Source: CAD feature listing. Evaluate the final solid. Frame: model axes, mm. Face numbers are marked on the shaded views. A direction names the side the tool comes from. Coordinates: 2 decimals unless noted, no trailing zeros. Write each loop counter-clockwise with the first axis right and the second up, starting at its lowest first coordinate (ties: lowest second). Pieces come first, ordered by that corner, then holes. Notation, with made-up numbers: (70.5, 63.25) - (87.5, 63.25) arc R21 cw to (87.5, 97.25) - close; hole circle Ø10 at (74.5, -18). An arc over 180 degrees is marked (long way). One line per item, written item: value.
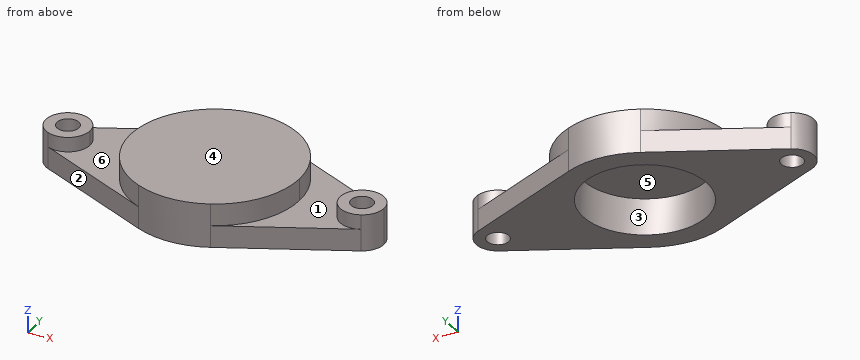
from build123d import *

# Parameters (mm, degrees)
F0_R     = 8.5
F1_DEPTH = 6
F2_DEPTH = 5
F0_R_2   = 1.5
F3_DEPTH = 5
F4_DEPTH = 3


with BuildPart() as f1:
    # F0 (on Top) → F1 (new body)
    with BuildSketch(Plane.XY):
        with BuildLine():
            ThreePointArc((4.8875, -10.4097235194), (9.7071172343, -6.1661880445), (11.5, 0))
            ThreePointArc((11.5, 0), (9.7071172343, 6.1661880445), (4.8875, 10.4097235194))
            ThreePointArc((4.8875, 10.4097235194), (0, 11.5), (-4.8875, 10.4097235194))
            ThreePointArc((-4.8875, 10.4097235194), (-11.5, 0), (-4.8875, -10.4097235194))
            ThreePointArc((-4.8875, -10.4097235194), (0, -11.5), (4.8875, -10.4097235194))
        make_face()
        Circle(F0_R, mode=Mode.SUBTRACT)
        Circle(F0_R)
    extrude(amount=F1_DEPTH)

    # F0 (on Top) → F2 (cut)
    with BuildSketch(Plane.XY):
        Circle(F0_R)
    extrude(amount=F2_DEPTH, mode=Mode.SUBTRACT)



with BuildPart() as f3:
    # F0 (on Top) → F3 (new body)
    with BuildSketch(Plane.XY):
        with BuildLine():
            ThreePointArc((-17, 0), (-18.3914292058, 2.5322914524), (-21.275, 2.7155800485))
            ThreePointArc((-21.275, 2.7155800485), (-23, 0), (-21.275, -2.7155800485))
            ThreePointArc((-21.275, -2.7155800485), (-18.3914292058, -2.5322914524), (-17, 0))
        make_face()
        with Locations((-20, 0)):
            Circle(F0_R_2, mode=Mode.SUBTRACT)
    extrude(amount=F3_DEPTH)


with BuildPart() as f3b:
    # F0 (on Top) → F3, piece 2 (new body)
    with BuildSketch(Plane.XY):
        with BuildLine():
            ThreePointArc((23, 0), (22.5322914524, 1.6085707942), (21.275, 2.7155800485))
            ThreePointArc((21.275, 2.7155800485), (17, 0), (21.275, -2.7155800485))
            ThreePointArc((21.275, -2.7155800485), (22.5322914524, -1.6085707942), (23, 0))
        make_face()
        with Locations((20, 0)):
            Circle(F0_R_2, mode=Mode.SUBTRACT)
    extrude(amount=F3_DEPTH)


with BuildPart() as f1_1:
    add(f1.part)

    add(f3.part)  # F4 merges F3

    add(f3b.part)  # F4 merges F3b
    # F0 (on Top) → F4 (join)
    with BuildSketch(Plane.XY):
        with BuildLine():
            ThreePointArc((-4.8875, -10.4097235194), (-11.5, 0), (-4.8875, 10.4097235194))
            Line((-4.8875, 10.4097235194), (-21.275, 2.7155800485))
            ThreePointArc((-21.275, 2.7155800485), (-18.3914292058, 2.5322914524), (-17, 0))
            ThreePointArc((-17, 0), (-18.3914292058, -2.5322914524), (-21.275, -2.7155800485))
            Line((-21.275, -2.7155800485), (-4.8875, -10.4097235194))
        make_face()
        with BuildLine():
            ThreePointArc((4.8875, 10.4097235194), (9.7071172343, 6.1661880445), (11.5, 0))
            ThreePointArc((11.5, 0), (9.7071172343, -6.1661880445), (4.8875, -10.4097235194))
            Line((4.8875, -10.4097235194), (21.275, -2.7155800485))
            ThreePointArc((21.275, -2.7155800485), (17, 0), (21.275, 2.7155800485))
            Line((21.275, 2.7155800485), (4.8875, 10.4097235194))
        make_face()
    extrude(amount=F4_DEPTH)


solid = f1_1.part
1) Material intervals for line 1 (Y direction, x = 20, z = 3.2); line 2 (Y direction, x = -5, z = 0.5); line 3 (X direction, y = 4.5, z = 0.4), sorted ascending.
Values found:
line 1: -3 to -1.5, 1.5 to 3
line 2: -10.36 to -6.87, 6.87 to 10.36
line 3: -17.47 to -7.21, 7.21 to 17.47
2) Section query D-D on y = 5.75. Output: boundary loops of the cut face in (x, z).
Values found:
outline: (-14.81, 0) - (-6.26, 0) - (-6.26, 5) - (6.26, 5) - (6.26, 0) - (14.81, 0) - (14.81, 3) - (9.96, 3) - (9.96, 6) - (-9.96, 6) - (-9.96, 3) - (-14.81, 3) - close
3) Section query C-C on x = -20. Output: boundary loops of the cut face in (y, z).
Values found:
outline: (-3.31, 0) - (-1.5, 0) - (-1.5, 5) - (-3, 5) - (-3, 3) - (-3.31, 3) - close; (1.5, 0) - (3.31, 0) - (3.31, 3) - (3, 3) - (3, 5) - (1.5, 5) - close
4) Section query B-B on x = 0. Output: boundary loops of the cut face in (y, z).
Values found:
outline: (-11.5, 0) - (-8.5, 0) - (-8.5, 5) - (8.5, 5) - (8.5, 0) - (11.5, 0) - (11.5, 6) - (-11.5, 6) - close
5) Section query A-A on z = 0.6. Output: boundary loops of the cut face in (x, y) (1 decimal), then the cut area to 3 significant figures.
Values found:
outline: (-21.3, -2.7) - (-4.9, -10.4) arc R11.5 ccw to (4.9, -10.4) - (21.3, -2.7) arc R3 ccw to (21.3, 2.7) - (4.9, 10.4) arc R11.5 ccw to (-4.9, 10.4) - (-21.3, 2.7) arc R3 ccw to start; hole circle Ø3 at (-20, 0); hole circle Ø17 at (0, 0); hole circle Ø3 at (20, 0)
area: 420 mm2
6) Draft query along Y for the marked faces 1, 2 and 3. Return one class per face: released by +Y, released by -Y, zero draft, split by the parting line, or undercut.
Values found:
face 1: zero draft
face 2: released by -Y
face 3: undercut
7) Contact query for flat-ended pins moving along their axis: P1, Ø3, axis at x = -19, y = 0, coming from the +Z side; P2, Ø2.5, axis at x = -20, y = 0, coming from the +Z side; P3, Ø4, axis at x = 4.5, y = -1.5, coming from the -Z side; P4, Ø1, axis at x = 5, z = 3, coming from the +Y side. Output: stop coordinate, or through.
Values found:
P1: z = 5
P2: through
P3: z = 5
P4: y = 10.58
8) Reachability of the marked faces 4, 5 and 6 from +Z, -Z, +X, -X, +Y, -Y: full face, straight path, thin tool, end or side. Return the list, or none.
Values found:
face 4: +Z, +X, -X, +Y, -Y
face 5: -Z
face 6: +Z
